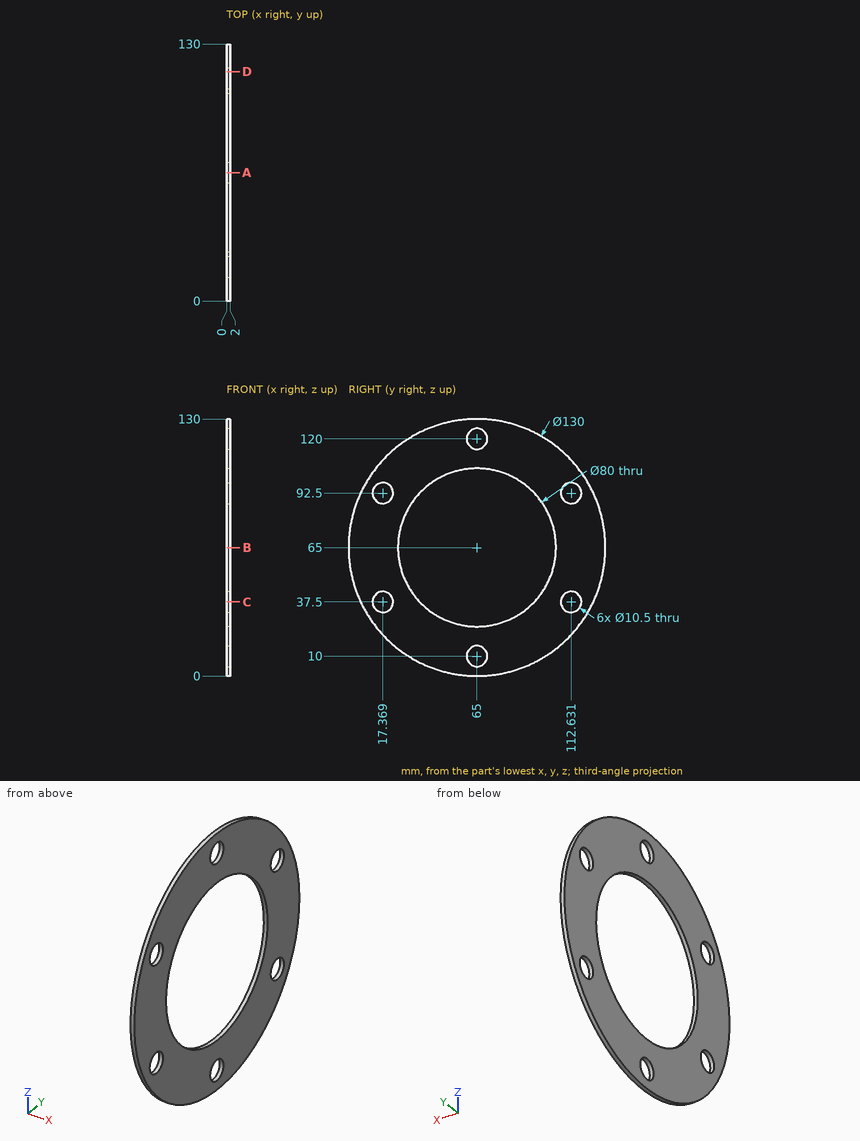
Here's the drawing with two shaded views (mm, measured from the low corner). I have some questions. Round coordinates to 2 decimals unless told otherwise and drop trailing zeros. Loops run counter-clockwise (first coordinate to the right, second up) from the corner with the lowest first, then second, coordinate; pieces in that order, holes last.
1. Will this pin go through, and if not, where does the flat tip stop? pin 1 (6.5 mm diameter, centred on y = 112.63, z = 92.5, fed in from +X).
Answers:
pin 1: passes through
2. Suppose I cut it at C-C, the plane z = 37.5. Please give me the cut outline in (x, y).
Answers:
outline: (0, 6.1) - (2, 6.1) - (2, 12.12) - (0, 12.12) - close; (0, 22.62) - (2, 22.62) - (2, 35.95) - (0, 35.95) - close; (0, 94.05) - (2, 94.05) - (2, 107.38) - (0, 107.38) - close; (0, 117.88) - (2, 117.88) - (2, 123.9) - (0, 123.9) - close
3. Suppose I cut it at A-A, the plane y = 65. Please give me the cut outline in (x, z).
Answers:
outline: (0, 0) - (2, 0) - (2, 4.75) - (0, 4.75) - close; (0, 15.25) - (2, 15.25) - (2, 25) - (0, 25) - close; (0, 105) - (2, 105) - (2, 114.75) - (0, 114.75) - close; (0, 125.25) - (2, 125.25) - (2, 130) - (0, 130) - close
4. Suppose I cut it at B-B, the plane z = 65. Please give me the cut outline in (x, y).
Answers:
outline: (0, 0) - (2, 0) - (2, 25) - (0, 25) - close; (0, 105) - (2, 105) - (2, 130) - (0, 130) - close
5. Suppose I cut it at D-D, the plane y = 116. Please give me the cut outline in (x, z).
Answers:
outline: (0, 24.7) - (2, 24.7) - (2, 33.47) - (0, 33.47) - close; (0, 41.53) - (2, 41.53) - (2, 88.47) - (0, 88.47) - close; (0, 96.53) - (2, 96.53) - (2, 105.3) - (0, 105.3) - close
6. If I drill on probe 1 along Y at (x, z) = (1.4, 37.5) (1 decimal); probe 2 along Z at (x, y) = (1.6, 17) (1 decimal); probe 3 along Y at (x, z) = (1.3, 89) (1 decimal), over which ranges is the centre line in solid material (lowest first)?
Answers:
probe 1: y = 6.1 to 12.1, 22.6 to 36, 94 to 107.4, 117.9 to 123.9
probe 2: z = 21.2 to 32.3, 42.7 to 87.3, 97.7 to 108.8
probe 3: y = 4.6 to 13.5, 21.3 to 33, 97 to 108.7, 116.5 to 125.4
